from build123d import *

# Parameters (mm, degrees)
EXTRUDE_1_DEPTH     = 3
CUT_EXTRUDE_1_DEPTH = 10
CUT_EXTRUDE_2_DEPTH = 10


with BuildPart() as part:
    # 草图1 → 凸台-拉伸1 (new body)
    with BuildSketch(Plane.XY):
        with BuildLine():
            Line((6.986719164, -53.161934409), (35.338837115, -34.396076908))
            ThreePointArc((35.338837115, -34.396076908), (36.622800273, -32.492523245), (36.184683625, -30.238608486))
            Line((36.184683625, -30.238608486), (-18.457077921, 52.316087899))
            ThreePointArc((-18.457077921, 52.316087899), (-20.360631584, 53.600051056), (-22.614546343, 53.161934409))
            Line((-22.614546343, 53.161934409), (-35.338837115, 44.739910071))
            ThreePointArc((-35.338837115, 44.739910071), (-36.370802739, 43.570865472), (-36.676585387, 42.041775777))
            Line((-36.676585387, 42.041775777), (-34.202704532, 4.349245051))
            ThreePointArc((-34.202704532, 4.349245051), (-34.051989945, 3.587476428), (-33.710802769, 2.889910923))
            Line((-33.710802769, 2.889910923), (2.829250742, -52.316087899))
            ThreePointArc((2.829250742, -52.316087899), (4.732804405, -53.600051056), (6.986719164, -53.161934409))
        make_face()
        with BuildLine():
            ThreePointArc((7.991481125, -42.903257428), (5.912746914, -42.480334173), (5.489823659, -44.559068384))
            ThreePointArc((5.489823659, -44.559068384), (7.56855787, -44.981991639), (7.991481125, -42.903257428))
        make_face(mode=Mode.SUBTRACT)
        with BuildLine():
            ThreePointArc((28.004740855, -29.65676978), (25.926006644, -29.233846525), (25.503083389, -31.312580736))
            ThreePointArc((25.503083389, -31.312580736), (27.5818176, -31.735503991), (28.004740855, -29.65676978))
        make_face(mode=Mode.SUBTRACT)
        with BuildLine():
            ThreePointArc((20.277623061, -17.982368271), (18.198888849, -17.559445016), (17.775965594, -19.638179227))
            ThreePointArc((17.775965594, -19.638179227), (19.854699805, -20.061102482), (20.277623061, -17.982368271))
        make_face(mode=Mode.SUBTRACT)
        with BuildLine():
            ThreePointArc((0.264363331, -31.228855919), (-1.81437088, -30.805932664), (-2.237294135, -32.884666875))
            ThreePointArc((-2.237294135, -32.884666875), (-0.158559924, -33.30759013), (0.264363331, -31.228855919))
        make_face(mode=Mode.SUBTRACT)
        with BuildLine():
            ThreePointArc((-7.732742612, -17.33474578), (-11.19729963, -16.629873689), (-11.902171722, -20.094430707))
            ThreePointArc((-11.902171722, -20.094430707), (-8.437614704, -20.799302799), (-7.732742612, -17.33474578))
        make_face(mode=Mode.SUBTRACT)
        with BuildLine():
            ThreePointArc((12.280517118, -4.088258133), (8.815960099, -3.383386041), (8.111088007, -6.84794306))
            ThreePointArc((8.111088007, -6.84794306), (11.575645026, -7.552815151), (12.280517118, -4.088258133))
        make_face(mode=Mode.SUBTRACT)
        with BuildLine():
            ThreePointArc((-20.97923026, 2.678513949), (-24.443787278, 3.383386041), (-25.14865937, -0.081170977))
            ThreePointArc((-25.14865937, -0.081170977), (-21.684102351, -0.786043069), (-20.97923026, 2.678513949))
        make_face(mode=Mode.SUBTRACT)
        with BuildLine():
            ThreePointArc((-0.96597053, 15.925001597), (-4.430527548, 16.629873689), (-5.13539964, 13.16531667))
            ThreePointArc((-5.13539964, 13.16531667), (-1.670842622, 12.460444578), (-0.96597053, 15.925001597))
        make_face(mode=Mode.SUBTRACT)
        with BuildLine():
            ThreePointArc((-5.315850745, 29.834747896), (-7.463876096, 30.271768593), (-7.900896793, 28.123743242))
            ThreePointArc((-7.900896793, 28.123743242), (-5.752871442, 27.686722545), (-5.315850745, 29.834747896))
        make_face(mode=Mode.SUBTRACT)
        with BuildLine():
            ThreePointArc((-15.446542758, 23.129389128), (-17.594568109, 23.566409825), (-18.031588806, 21.418384473))
            ThreePointArc((-18.031588806, 21.418384473), (-15.883563455, 20.981363776), (-15.446542758, 23.129389128))
        make_face(mode=Mode.SUBTRACT)
        with BuildLine():
            ThreePointArc((-16.354590451, 46.512464337), (-18.502615803, 46.949485034), (-18.9396365, 44.801459683))
            ThreePointArc((-18.9396365, 44.801459683), (-16.791611148, 44.364438986), (-16.354590451, 46.512464337))
        make_face(mode=Mode.SUBTRACT)
        with BuildLine():
            ThreePointArc((-25.527334494, 40.441157499), (-27.675359845, 40.878178196), (-28.112380542, 38.730152845))
            ThreePointArc((-28.112380542, 38.730152845), (-25.964355191, 38.293132148), (-25.527334494, 40.441157499))
        make_face(mode=Mode.SUBTRACT)
    extrude(amount=EXTRUDE_1_DEPTH)

    # 草图2 → 切除-拉伸1 (cut)
    with BuildSketch(Plane.XY.offset(3)):
        Polygon((-17.618504331, 51.049141407), (-36.449708749, 38.585039103), (-39.080293109, 42.559418534), (-20.249088692, 55.023520838), align=None)
        Polygon((22.294234295, -9.252428783), (-11.061198588, -31.329908196), (5.024024644, -55.632029551), (41.740524867, -31.329908196), align=None)
    extrude(amount=-CUT_EXTRUDE_1_DEPTH, mode=Mode.SUBTRACT)

    # 草图3 → 切除-拉伸2 (cut)
    with BuildSketch(Plane.XY.offset(3)):
        Polygon((-13.268946529, -27.994364908), (20.086486354, -5.916885495), (39.339377522, -11.508432246), (-14.131394495, -36.930591808), align=None)
    extrude(amount=-CUT_EXTRUDE_2_DEPTH, mode=Mode.SUBTRACT)


solid = part.part
Here's how the part is built. I have some questions about the finished solid (model axes, mm). Coordinates: 2 decimals unless noted, no trailing zeros. Loops run counter-clockwise (first coordinate to the right, second up) from the corner with the lowest first, then second, coordinate; pieces in that order, holes last.
1. Imagine slicing it at C-C, the plane y = 35. Please give me the cut outline in (x, z).
2. For P1, Ø3, axis at x = -26.82, y = 39.59, coming from the -Z side, with a flat end and sliding along its axis, tell me the tip position at first contact or that it passes through.
3. Imagine slicing it at D-D, the plane x = -2. Please give me the cut outline in (y, z).
4. Imagine slicing it at B-B, the plane z = 1.6. Count the separate pieces of the cut face and the enclosed holes in it, and give its area (3 significant figures).
5. I need wall thicknesses on L1, parallel to Y at x = -18, z = 1.95; L2, parallel to X at y = -3.5, z = 1.9; L3, parallel to X at y = 47, z = 2.6. Which ranges of each line are inside material? Lowest first, please.
6. Imagine slicing it at A-A, the plane x = 9. Please give me the cut outline in (y, z), and give its area (3 significant figures).
7. If we mould it in two halves opening along Y, with no side actions, what happens to faces 1 (the cylindrical face through (-34.055, 3.598, 1.479)), 2 (the cylindrical face through (-27.375, 41.033, 1.479)), 3 (the flat face through (-26.902, 44.904, 1.521))? For each: pulls with the +Y half, pulls with the -Y half, needs draft (parallel to the pull), parting line crosses it, or undercut.
Taken from the geometry:
1. outline: (-36.21, 0) - (-7, 0) - (-7, 3) - (-36.21, 3) - close
2. P1: passes through
3. outline: (-20.54, 0) - (12.28, 0) - (12.28, 3) - (-20.54, 3) - close; (16.81, 0) - (27.45, 0) - (27.45, 3) - (16.81, 3) - close
4. separate pieces: 1
4. enclosed holes: 8
4. area: 2,360 mm2
5. L1: y = -20.85 to 21.37, 23.18 to 44.15, 47.17 to 50.8
5. L2: x = -29.48 to 8.65, 11.74 to 18.49
5. L3: x = -23.74 to -18.42, -16.87 to -14.94
6. outline: (-13.25, 0) - (-7.66, 0) - (-7.66, 3) - (-13.25, 3) - close; (-3.27, 0) - (10.83, 0) - (10.83, 3) - (-3.27, 3) - close
6. area: 59.1 mm2
7. face 1: pulls with the -Y half
7. face 2: undercut
7. face 3: pulls with the +Y half
